Design review of the part built by this model. Coordinates are the model's own, in mm. Face numbers are marked on the shaded views. A direction names the side the tool comes from. Coordinates: 2 decimals unless noted, no trailing zeros. Loops run counter-clockwise (first coordinate to the right, second up) from the corner with the lowest first, then second, coordinate; pieces in that order, holes last. Notation, with made-up numbers: (65.5, -35) -> (97.5, -35) arc R19 ccw to (97.5, -9) -> close; hole circle Ø2 at (61.5, 31). An arc over 180 degrees is marked (long way). Answer in a Markdown table with one row per item.
Autodesk Inventor part; units mm, degrees
ref_plane "YZ Plane" through (0, 0, 0) normal (1, 0, 0) x (0, 1, 0)
ref_plane "XZ Plane" through (0, 0, 0) normal (0, 1, 0) x (-1, 0, 0)
ref_plane "XY Plane" through (0, 0, 0) normal (0, 0, 1) x (1, 0, 0)
sketch "Sketch1" plane through (0, 0, 0) normal (0, 1, 0) x (-1, 0, 0)
  line L0 (0, 0) -> (225, 0)
  line L1 (225, 0) -> (225, -150)
  line L2 (225, -150) -> (0, -150)
  line L3 (0, -150) -> (0, 0)
  dimension "d0" = 225
  dimension "d1" = 150
extrude "Extrusion1" add sketch "Sketch1" along normal blind 10
sketch "Sketch2" plane through (-225, 0, 0) normal (0, 0, 1) x (1, 0, 0)
  line L0 (0, 0) -> (0, 10)
  line L1 (225, 0) -> (225, 10)
  line L2 (0, 7.5) -> (225, 7.5)
  line L3 (225, 7.5) -> (225, 2.5)
  line L4 (225, 2.5) -> (0, 2.5)
  line L5 (0, 2.5) -> (0, 7.5)
  line L6 (225, 7.5) -> (210, 7.5)
  line L7 (210, 7.5) -> (210, 2.5)
  line L8 (210, 2.5) -> (225, 2.5)
  line L9 (225, 2.5) -> (225, 7.5)
  line L10 (0, 7.5) -> (15, 7.5)
  line L11 (15, 7.5) -> (15, 2.5)
  line L12 (15, 2.5) -> (0, 2.5)
  line L13 (0, 2.5) -> (0, 7.5)
  dimension "d4" = 5
  dimension "d5" = 15
  dimension "d6" = 5
  dimension "d7" = 15
  dimension "d8" = 5
sketch "Sketch3" plane through (0, 0, 0) normal (1, 0, 0) x (0, 0, -1)
  line L0 (0, 0) -> (0, 10)
  line L1 (0, 7.5) -> (150, 7.5)
  line L2 (150, 7.5) -> (150, 2.5)
  line L3 (150, 2.5) -> (0, 2.5)
  line L4 (0, 2.5) -> (0, 7.5)
  line L5 (0, 7.5) -> (15, 7.5)
  line L6 (15, 7.5) -> (15, 2.5)
  line L7 (15, 2.5) -> (0, 2.5)
  line L8 (0, 2.5) -> (0, 7.5)
  line L9 (150, 7.5) -> (135, 7.5)
  line L10 (135, 7.5) -> (135, 2.5)
  line L11 (135, 2.5) -> (150, 2.5)
  line L12 (150, 2.5) -> (150, 7.5)
  dimension "d9" = 150
  dimension "d10" = 5
  dimension "d11" = 15
  dimension "d12" = 5
  dimension "d13" = 15
  dimension "d14" = 5
extrude "Extrusion2" add sketch "Sketch2" along normal blind 25 contours L11 L2 L7 L4
extrude "Extrusion3" cut sketch "Sketch3" against normal blind 25 contours L6 L1 L10 L3
sketch "Sketch4" plane through (0, 0, 0) normal (0, -1, 0) x (1, 0, 0)
  line L0 (-225, -150) -> (-225, 0)
  line L1 (-225, -50) -> (-215, -50)
  line L2 (-215, -50) -> (-215, -80)
  line L3 (-215, -80) -> (-225, -80)
  line L4 (-225, -80) -> (-225, -50)
  line L5 (-50, -150) -> (-155, -150)
  line L6 (-155, -150) -> (-155, -140)
  line L7 (-155, -140) -> (-50, -140)
  line L8 (-50, -140) -> (-50, -150)
  point P0 (0, 0)
  dimension "d19" = 10
  dimension "d20" = 30
  dimension "d21" = 105
  dimension "d22" = 10
extrude "Extrusion4" add sketch "Sketch4" along normal blind 10
properties part number "TSU_MF_Floor"
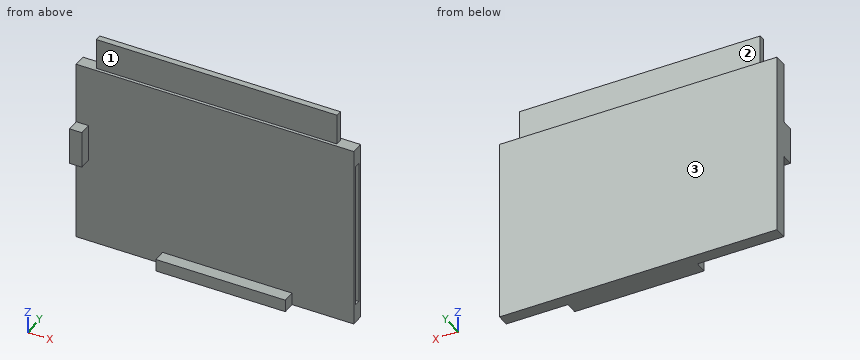
(1) Take a section at A-A on y = -7. Give the boundary of the cut face in (x, z).
Evaluation:
| item | result |
|---|---|
| outline | (-225, -80) -> (-215, -80) -> (-215, -50) -> (-225, -50) -> close; (-155, -150) -> (-50, -150) -> (-50, -140) -> (-155, -140) -> close |
(2) Take a section at D-D on x = -54. Give the boundary of the cut face in (y, z).
Evaluation:
| item | result |
|---|---|
| outline | (-10, -150) -> (10, -150) -> (10, 0) -> (7.5, 0) -> (7.5, 25) -> (2.5, 25) -> (2.5, 0) -> (0, 0) -> (0, -140) -> (-10, -140) -> close |
(3) Tool access review of the marked faces 1, 2 and 3: name each direction out of +Z, -Z, +X, -X, +Y, -Y from which nothing blocks a thin tool from reaching the whole face with its end or side.
Evaluation:
| item | result |
|---|---|
| face 1 | +Z, +X, -X, -Y |
| face 2 | +Z, +X, -X, +Y |
| face 3 | +Z, -Z, +X, -X, +Y |
(4) To check wall thickness, follow probe 1 along X at (y, z) = (6, -83.5); probe 2 along Y at (x, z) = (-76, -49); probe 3 along Z at (x, y) = (-99.5, 0.75). State the ranges of each line that lie inside material, in increasing order.
Evaluation:
| item | result |
|---|---|
| probe 1 | x = -225 to -25 |
| probe 2 | y = 0 to 10 |
| probe 3 | z = -150 to 0 |
(5) Take a section at C-C on z = -42. Give the boundary of the cut face in (x, y), and give its area (4 significant figures).
Evaluation:
| item | result |
|---|---|
| outline | (-225, 0) -> (0, 0) -> (0, 2.5) -> (-25, 2.5) -> (-25, 7.5) -> (0, 7.5) -> (0, 10) -> (-225, 10) -> close |
| area | 2,125 mm² |
(6) For pin 1 (12.5 mm diameter, centred on x = -113, z = 7, fed in from -Y); pin 2 (5 mm diameter, centred on y = -3, z = -144, fed in from +X); pin 3 (12 mm diameter, centred on x = -144.5, z = -98.5, fed in from -Y), all flat-tipped, find the tip position at first contact; note any pin that passes through.
Evaluation:
| item | result |
|---|---|
| pin 1 | stops at y = 2.5 |
| pin 2 | stops at x = -50 |
| pin 3 | stops at y = 0 |
(7) Take a section at B-B on x = -20.5. Give the boundary of the cut face in (y, z).
Evaluation:
| item | result |
|---|---|
| outline | (0, -150) -> (10, -150) -> (10, 0) -> (7.5, 0) -> (7.5, 25) -> (2.5, 25) -> (2.5, 0) -> (0, 0) -> close; hole (2.5, -135) -> (7.5, -135) -> (7.5, -15) -> (2.5, -15) -> close |
